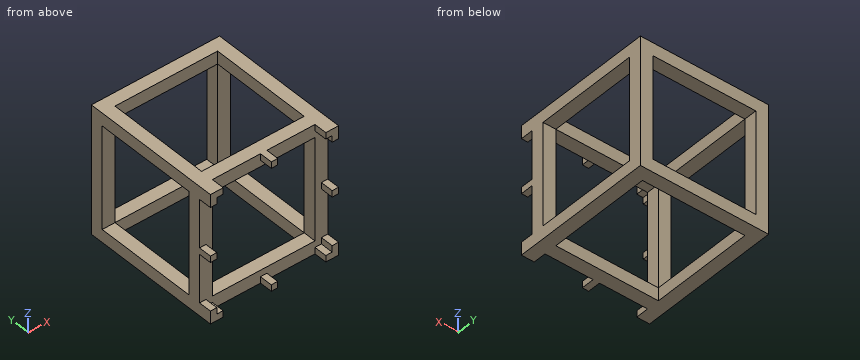
Autodesk Inventor part; units mm, degrees
ref_plane "YZ Plane" through (0, 0, 0) normal (1, 0, 0) x (0, 1, 0)
ref_plane "XZ Plane" through (0, 0, 0) normal (0, 1, 0) x (-1, 0, 0)
ref_plane "XY Plane" through (0, 0, 0) normal (0, 0, 1) x (1, 0, 0)
sketch "Sketch1" plane through (0, 0, 0) normal (0, 1, 0) x (-1, 0, 0)
  line L0 (50, -50) -> (-50, -50)
  line L1 (-50, -50) -> (-50, 50)
  line L2 (-50, 50) -> (50, 50)
  line L3 (50, 50) -> (50, -50)
  point P0 (0, 0)
  dimension "d0" = 100
  dimension "d1" = 100
  dimension "d2" = 50
  dimension "d3" = 50
extrude "Extrusion1" add sketch "Sketch1" along normal blind 100
sketch "Sketch2" plane through (-50, 0, 50) normal (0, 0, 1) x (1, 0, 0)
  line L0 (10, 90) -> (90, 90)
  line L1 (90, 90) -> (90, 10)
  line L2 (90, 10) -> (10, 10)
  line L3 (10, 10) -> (10, 90)
  line L4 (100, 0) -> (0, 0)
  line L5 (100, 0) -> (100, 100)
  point P0 (50, 0)
  dimension "d6" = 80
  dimension "d7" = 10
  dimension "d8" = 80
  dimension "d9" = 10
extrude "Extrusion2" cut sketch "Sketch2" against normal blind 100
sketch "Sketch3" plane through (50, 0, 50) normal (1, 0, 0) x (0, 0, -1)
  line L0 (10, 90) -> (90, 90)
  line L1 (90, 90) -> (90, 10)
  line L2 (90, 10) -> (10, 10)
  line L3 (10, 10) -> (10, 90)
  line L4 (0, 100) -> (100, 100)
  line L5 (100, 0) -> (100, 100)
  point P0 (50, 0)
  dimension "d12" = 80
  dimension "d13" = 10
  dimension "d14" = 80
  dimension "d15" = 10
extrude "Extrusion3" cut sketch "Sketch3" against normal blind 100
sketch "Sketch4" plane through (0, 100, 0) normal (0, 1, 0) x (1, 0, 0)
  line L0 (-40, -50) -> (-40, -40)
  line L1 (50, 40) -> (40, 40)
  line L2 (-40, -40) -> (40, -40)
  line L3 (40, -40) -> (40, 40)
  line L4 (40, 40) -> (-40, 40)
  line L5 (-40, 40) -> (-40, -40)
  point P0 (0, 0)
extrude "Extrusion4" cut sketch "Sketch4" against normal blind 100
sketch "Sketch9" plane through (0, 0, 0) normal (0, -1, 0) x (1, 0, 0)
  line L0 (50, 0.0049) -> (45, 0.0049)
  line L1 (45, 0.0049) -> (45, -2.4951)
  line L2 (45, -2.4951) -> (50, -2.4951)
  line L3 (50, -2.4951) -> (50, 0.0049)
  line L4 (40, 40) -> (40, -40)
  point P0 (0, 0)
  dimension "d40" = 5
  dimension "d41" = 5
  dimension "d42" = 2.5
sketch "Sketch10" plane through (0, 0, 0) normal (0, -1, 0) x (1, 0, 0)
  line L0 (50, -40) -> (50, 40)
  line L1 (50, 0) -> (45, 0)
  line L2 (45, 0) -> (45, 2.5)
  line L3 (45, 2.5) -> (50, 2.5)
  line L4 (50, 2.5) -> (50, 0)
  line L5 (40, 40) -> (40, -40)
  point P0 (0, 0)
  dimension "d43" = 2.5
  dimension "d44" = 5
extrude "Extrusion9" add sketch "Sketch9" along normal blind 10
extrude "Extrusion10" add sketch "Sketch10" along normal blind 10
mirror "Mirror3" about plane through (0, 0, 0) normal (1, 0, 0) of "Extrusion9", "Extrusion10"
sketch "Sketch11" plane through (0, 0, 0) normal (0, -1, 0) x (1, 0, 0)
  line L0 (-40, -50) -> (40, -50)
  line L1 (0, -50) -> (-2.5, -50)
  line L2 (-2.5, -50) -> (-2.5, -45)
  line L3 (-2.5, -45) -> (0, -45)
  line L4 (0, -45) -> (0, -50)
  line L5 (40, -40) -> (-40, -40)
  point P0 (0, 0)
  dimension "d49" = 5
  dimension "d50" = 2.5
sketch "Sketch12" plane through (0, 0, 0) normal (0, -1, 0) x (1, 0, 0)
  line L0 (-40, -50) -> (40, -50)
  line L1 (0, -50) -> (2.5, -50)
  line L2 (2.5, -50) -> (2.5, -45)
  line L3 (2.5, -45) -> (0, -45)
  line L4 (0, -45) -> (0, -50)
  line L5 (40, -40) -> (-40, -40)
  point P0 (0, 0)
  dimension "d51" = 5
  dimension "d52" = 2.5
extrude "Extrusion11" add sketch "Sketch11" along normal blind 10
extrude "Extrusion12" add sketch "Sketch12" along normal blind 10
mirror "Mirror4" about plane through (0, 0, 0) normal (0, 0, 1) of "Extrusion11", "Extrusion12"
sketch "Sketch13" plane through (0, 0, 0) normal (0, -1, 0) x (1, 0, 0)
  line L0 (50, -40) -> (50, 40)
  line L1 (50, -50) -> (-50, -50)
  line L2 (50, -40) -> (45, -40)
  line L3 (45, -40) -> (45, -50)
  line L4 (45, -50) -> (50, -50)
  line L5 (50, -50) -> (50, -40)
  line L6 (40, 40) -> (40, -40)
  line L7 (45, -45) -> (40, -45)
  line L8 (40, -45) -> (40, -50)
  line L9 (40, -50) -> (45, -50)
  line L10 (45, -50) -> (45, -45)
  point P0 (0, 0)
  dimension "d57" = 5
extrude "Extrusion13" add sketch "Sketch13" along normal blind 10
mirror "Mirror5" about plane through (0, 0, 0) normal (0, 0, 1) of "Extrusion13"
mirror "Mirror6" about plane through (0, 0, 0) normal (1, 0, 0) of "Extrusion13"
mirror "Mirror7" about plane through (0, 0, 0) normal (0, 0, 1) of "Extrusion13", "Mirror6"
properties part number "Kens_cube_of_fun_design_withpegs_spencermical"
Source: CAD feature listing. Evaluate the final solid. Frame: model axes, mm. Coordinates: 2 decimals unless noted, no trailing zeros. Write each loop counter-clockwise with the first axis right and the second up, starting at its lowest first coordinate (ties: lowest second). Pieces come first, ordered by that corner, then holes. Notation, with made-up numbers: M 16,16.25 L 39,16.25 A17 ccw 39,23.25 Z; hole C 39,-11.75 d10. An arc over 180 degrees is marked long. Use a Markdown table: item, result.
1) Section A-A, the plane x = 10. Output: boundary loops of the cut face in (y, z), then the cut area to 3 significant figures.
Conclusion:
| item | result |
|---|---|
| outline | M 0,-50 L 10,-50 L 10,-40 L 0,-40 Z; M 0,40 L 10,40 L 10,50 L 0,50 Z; M 90,-50 L 100,-50 L 100,-40 L 90,-40 Z; M 90,40 L 100,40 L 100,50 L 90,50 Z |
| area | 400 mm^2 |
2) Section B-B, the plane z = -6.5. Output: boundary loops of the cut face in (x, y), then the cut area to 3 significant figures.
Conclusion:
| item | result |
|---|---|
| outline | M -50,0 L -40,0 L -40,10 L -50,10 Z; M -50,90 L -40,90 L -40,100 L -50,100 Z; M 40,0 L 50,0 L 50,10 L 40,10 Z; M 40,90 L 50,90 L 50,100 L 40,100 Z |
| area | 400 mm^2 |
3) Ray query, L1, parallel to Z at x = 17, y = 1; L2, parallel to Y at x = -6.5, z = 42. Return the intervals inside material, ascending.
Conclusion:
| item | result |
|---|---|
| L1 | z = -50 to -40, 40 to 50 |
| L2 | y = 0 to 10, 90 to 100 |
4) Section C-C, the plane y = 93.5. Output: boundary loops of the cut face in (x, z).
Conclusion:
| item | result |
|---|---|
| outline | M -50,-50 L 50,-50 L 50,50 L -50,50 Z; hole M -40,-40 L 40,-40 L 40,40 L -40,40 Z |
5) First-contact query: pin 1 Ø11 at (x, z) = (44, 14.5) entering from -Y. Flat tip, straight axial feed; report the tip coordinate or a pass-through.
Conclusion:
| item | result |
|---|---|
| pin 1 | stops at y = 0 |
